```python
from build123d import *

# Parameters (mm, degrees)
F0_W     = 25
F0_H     = 25
F1_DEPTH = 2
F3_DEPTH = 1.5
F4_W     = 27.374725
F4_H     = 28.161746
F5_DEPTH = 1
F6_R     = 1


with BuildPart() as f1:
    # F0 (on Top) → F1 (new body)
    with BuildSketch(Plane.XY):
        Rectangle(F0_W, F0_H)
    extrude(amount=F1_DEPTH)

    # F2 (on face) → F3 (cut)
    with BuildSketch(Plane.XY.offset(2)):
        with BuildLine():
            Line((12.5, -10.5), (12.5, 12.5))
            Line((12.5, 12.5), (-10.5, 12.5))
            ThreePointArc((-10.5, 12.5), (-3.763456, -3.763456), (12.5, -10.5))
        make_face()
    extrude(amount=-F3_DEPTH, mode=Mode.SUBTRACT)

    # F4 (on face) → F5 (cut)
    with BuildSketch(Plane.XY.offset(0.5)):
        with Locations((2.187362, 2.580873)):
            Rectangle(F4_W, F4_H)
    extrude(amount=F5_DEPTH, mode=Mode.SUBTRACT)

    # F6
    f6_edges = [f1.edges().sort_by_distance(p)[0] for p in [
        (-12.5, -12.5, 1),
    ]]
    fillet(f6_edges, radius=F6_R)


solid = f1.part
```
Design review of the part built by this model. Coordinates are the model's own, in mm. A direction names the side the tool comes from. Give positions to 0.01 mm unless a question says otherwise; leave off trailing zeros. Order: outer loops, then holes, each group sorted by start corner. A loop starts at its lowest first (then second) coordinate and runs counter-clockwise, first axis right, second up. Notation, with made-up numbers: (61.25, 89) -> (112.25, 89) arc R23 cw to (112.25, 106) -> close; hole circle Ø7 at (-4.5, -9.5). An arc over 180 degrees is marked (long way). Write each question's results on one line, items separated by ' | '. Start each with the question number.
Q1. Mouldability with a two-part tool opening along Z and no side actions: class faces 1 (the flat face through (0, 1, 0.5)), 2 (the cylindrical face through (-12.215, -12.199, 1.014)), 3 (the flat face through (-6, -6, 2)) as +Z half, -Z half, draft (parallel to the pull), parting line (faces both ways), or undercut.
Q2. Machinability: for faces 4 (the cylindrical face through (-3.941, -3.584, 1.754)), 5 (the flat face through (12.5, -1.9, 0.3)), 6 (the flat face through (0, -11.5, 1)), which of the approach directions +Z, -Z, +X, -X, +Y, -Y give a long, thin tool a straight path to every point of the face, cutting with its end or side? Answer none if there is none.
Q3. For pin 1 (1 mm diameter, centred on x = 8, z = 1.5, fed in from +Y); pin 2 (1 mm diameter, centred on x = 6.5, y = -1, fed in from +Z); pin 3 (0.5 mm diameter, centred on y = -3, z = 1, fed in from +X), all flat-tipped, find the tip position at first contact; note any pin that passes through.
Q4. Add section B-B on x = 8.5. Give the boundary of the cut face in (y, z).
Q5. Wall thickness on L1, parallel to Z at x = -5.5, y = -11; L2, parallel to X at y = -5.25, z = 1.45; L3, parallel to Z at x = 5.5, y = 2.5: over which ranges is each line inside the solid? List them lowest first. Write a range as from..to.
Q6. Add section A-A on y = -11. Give the boundary of the cut face in (x, z), and give its area (3 significant figures).
Found:
1) face 1: undercut | face 2: draft | face 3: +Z half
2) face 4: +Z, +X, +Y | face 5: +Z, -Z, +X, +Y, -Y | face 6: +X, +Y
3) pin 1: stops at y = -9.95 | pin 2: stops at z = 0.5 | pin 3: stops at x = -11.5
4) outline: (-12.5, 0) -> (12.5, 0) -> (12.5, 0.5) -> (-11.5, 0.5) -> (-11.5, 1.5) -> (-10.15, 1.5) -> (-10.15, 2) -> (-12.5, 2) -> close
5) L1: z = 0..0.5, 1.5..2 | L2: x = -12.5..-11.5 | L3: z = 0..0.5
6) outline: (-12.5, 0) -> (12.5, 0) -> (12.5, 0.5) -> (-11.5, 0.5) -> (-11.5, 1.5) -> (12.5, 1.5) -> (12.5, 2) -> (-12.5, 2) -> close | area: 26.0 mm2
